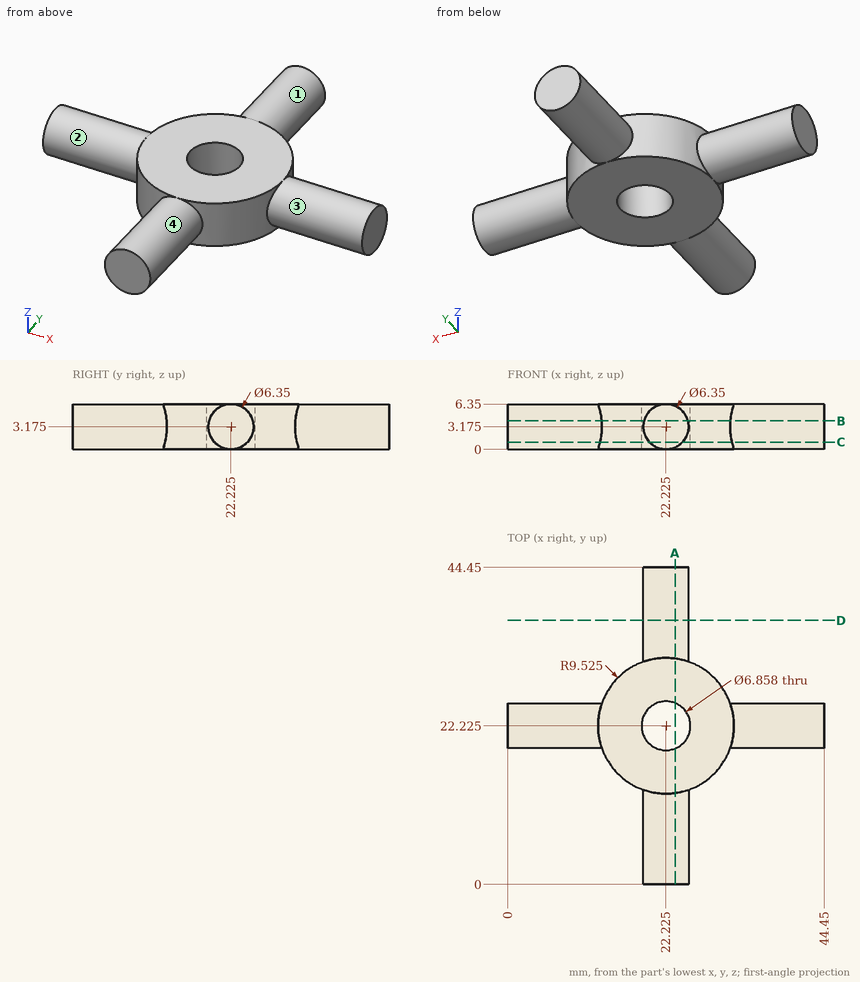
The figure shows three views and two pictorial views of one solid part (mm, origin at its lowest corner). Answer the questions. A direction names the side the tool comes from. Give positions to 0.01 mm unless a question says otherwise; leave off trailing zeros. Order: outer loops, then holes, each group sorted by start corner. A loop starts at its lowest first (then second) coordinate and runs counter-clockwise, first axis right, second up. Notation, with made-up numbers: M -26,32.5 L 10,32.5 A30 ccw 10,55.5 Z; hole C -23,55 d6. An arc over 180 degrees is marked long. Return JSON: item names as keys, results as strings.
Q1. Find section C-C, the plane z = 1. Write down the section's boundary in (x, y) (3 decimals).
Answer below:
{"outline": "M 0,19.912 L 12.985,19.912 A9.525 ccw 19.912,12.985 L 19.912,0 L 24.538,0 L 24.538,12.985 A9.525 ccw 31.465,19.912 L 44.45,19.912 L 44.45,24.538 L 31.465,24.538 A9.525 ccw 24.538,31.465 L 24.538,44.45 L 19.912,44.45 L 19.912,31.465 A9.525 ccw 12.985,24.538 L 0,24.538 Z; hole C 22.225,22.225 d6.858"}
Q2. Find section A-A, the plane x = 23.5. Write down the section's boundary in (y, z).
Answer below:
{"outline": "M 0,0.27 L 12.79,0.27 L 12.79,0 L 19.04,0 L 19.04,6.35 L 12.79,6.35 L 12.79,6.08 L 0,6.08 Z; M 25.41,0 L 31.66,0 L 31.66,0.27 L 44.45,0.27 L 44.45,6.08 L 31.66,6.08 L 31.66,6.35 L 25.41,6.35 Z"}
Q3. Each of these flat-tipped pins is pushed along its axis until it touches: pin 1 (2 mm diameter, centred on y = 39, z = 2, fed in from -X); pin 2 (4 mm diameter, centred on x = 36, y = 26, fed in from -Z); pin 3 (1 mm diameter, centred on x = 15, z = 1, fed in from -Y). Where does it stop, or does it pass through?
Answer below:
{"pin 1": "stops at x = 19.05", "pin 2": "stops at z = 0.54", "pin 3": "stops at y = 15.48"}
Q4. Which of the six approach directions +Z, -Z, +X, -X, +Y, -Y give full straight-line access (tool end or side, diameter ignored) to the marked faces 1, 2, 3 and 4?
Answer below:
{"face 1": "+Y", "face 2": "-X", "face 3": "+X", "face 4": "-Y"}
Q5. Find section D-D, the plane y = 37. Write down the section's boundary in (x, z) (3 decimals).
Answer below:
{"outline": "C 22.225,3.175 d6.35"}
Q6. Find section B-B, the plane z = 4. Write down the section's boundary in (x, y) (3 decimals).
Answer below:
{"outline": "M 0,19.159 L 13.207,19.159 A9.525 ccw 19.159,13.207 L 19.159,0 L 25.291,0 L 25.291,13.207 A9.525 ccw 31.243,19.159 L 44.45,19.159 L 44.45,25.291 L 31.243,25.291 A9.525 ccw 25.291,31.243 L 25.291,44.45 L 19.159,44.45 L 19.159,31.243 A9.525 ccw 13.207,25.291 L 0,25.291 Z; hole C 22.225,22.225 d6.858"}
Q7. Find the intervals of material crossed by line 1 along X through (y, z) = (25, 2); line 2 along X through (y, z) = (21, 5); line 3 along X through (y, z) = (2.5, 5.75), in increasing order. Write a range as [from, to].
Answer below:
{"line 1": "x = [0, 20.21], [24.24, 44.45]", "line 2": "x = [0, 19.02], [25.43, 44.45]", "line 3": "x = [20.37, 24.08]"}
